Here's the drawing with two shaded views (mm, measured from the low corner). I have some questions. A direction names the side the tool comes from. Give positions to 0.01 mm unless a question says otherwise; leave off trailing zeros. Loops run counter-clockwise (first coordinate to the right, second up) from the corner with the lowest first, then second, coordinate; pieces in that order, holes last. Notation, with made-up numbers: (19.25, -15) - (66.25, -15) arc R24 ccw to (66.25, 16) - close; hole circle Ø8 at (61, 40). An arc over 180 degrees is marked (long way). Answer as a JSON object with one key per item and string values. Group by question number.
Item 1: Suppose I cut it at D-D on x = 45.5. Write out the boundary of the cut face in (y, z), and give its area (3 significant figures).
Item 2: Suppose I cut it at B-B on y = 31. Write out the boundary of the cut face in (x, z), and give its area (3 significant figures).
Item 3: Suppose I cut it at C-C on x = 23.5. Write out the boundary of the cut face in (y, z), and give its area (3 significant figures).
Item 4: Which directions (+Z, -Z, +X, -X, +Y, -Y) give clear straight access to the entire face, cutting with the end or side of a thin tool? Please do the marked faces 1 and 2.
Item 5: Please list where these lines run through material, in increasing order: L1, parallel to Y at x = 27, z = 145; L2, parallel to Y at x = 16, z = 14; L3, parallel to X at y = 7.5, z = 107.
Item 6: Will these pins go through, and if not, where does the flat tip stop? pin 1 (14.5 mm diameter, centred on y = 19.05, z = 145.38, fed in from -X); pin 2 (11 mm diameter, centred on x = 51.5, y = 35, fed in from +Z); pin 3 (21 mm diameter, centred on x = 9, z = 45.5, fed in from -Y).
Item 7: Suppose I cut it at A-A on z = 145.38. Write out the boundary of the cut face in (x, y).
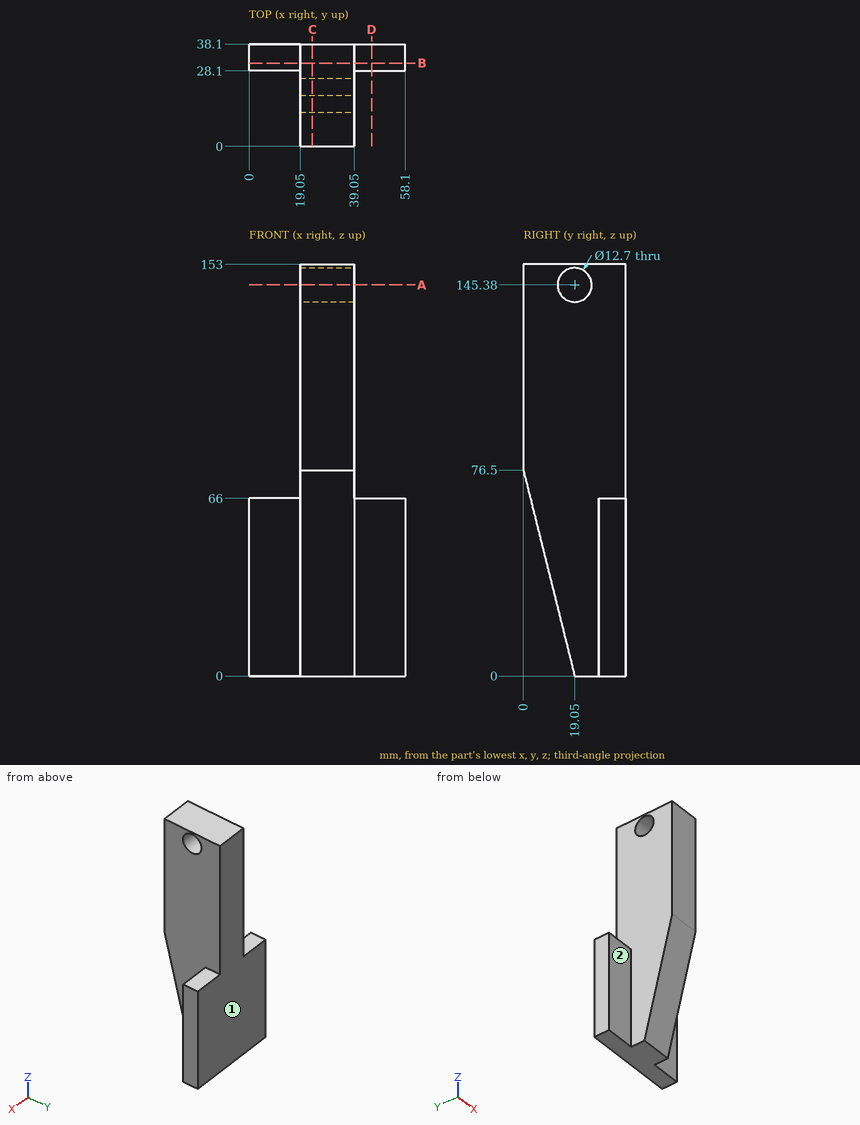
Worked out:
{
 "1": {"outline": "(28.1, 0) - (38.1, 0) - (38.1, 66) - (28.1, 66) - close", "area": "660 mm2"},
 "2": {"outline": "(0, 0) - (58.1, 0) - (58.1, 66) - (39.05, 66) - (39.05, 153) - (19.05, 153) - (19.05, 66) - (0, 66) - close", "area": "5,570 mm2"},
 "3": {"outline": "(0, 76.5) - (19.05, 0) - (38.1, 0) - (38.1, 153) - (0, 153) - close; hole circle Ø12.7 at (19.05, 145.38)", "area": "4,970 mm2"},
 "4": {"face 1": "+Z, -Z, +X, -X, +Y", "face 2": "+Z, -Z, -X, -Y"},
 "5": {"L1": "y = 0 to 12.71, 25.39 to 38.1", "L2": "y = 28.1 to 38.1", "L3": "x = 19.05 to 39.05"},
 "6": {"pin 1": "stops at x = 19.05", "pin 2": "stops at z = 66", "pin 3": "stops at y = 6.96"},
 "7": {"outline": "(19.05, 0) - (39.05, 0) - (39.05, 12.7) - (19.05, 12.7) - close; (19.05, 25.4) - (39.05, 25.4) - (39.05, 38.1) - (19.05, 38.1) - close"}
}
